Print and shaded views of the part. All mm, measured from the part's lowest x, y and z. A direction names the side the tool comes from. Round coordinates to 2 decimals unless told otherwise and drop trailing zeros. Order: outer loops, then holes, each group sorted by start corner. A loop starts at its lowest first (then second) coordinate and runs counter-clockwise, first axis right, second up. Notation, with made-up numbers: M -17.75,-14 L 18.25,-14 A17 cw 18.25,13 Z; hole C -30,40.5 d1. An arc over 180 degrees is marked long. Use CSV: the item, a comma, the result in double quotes.
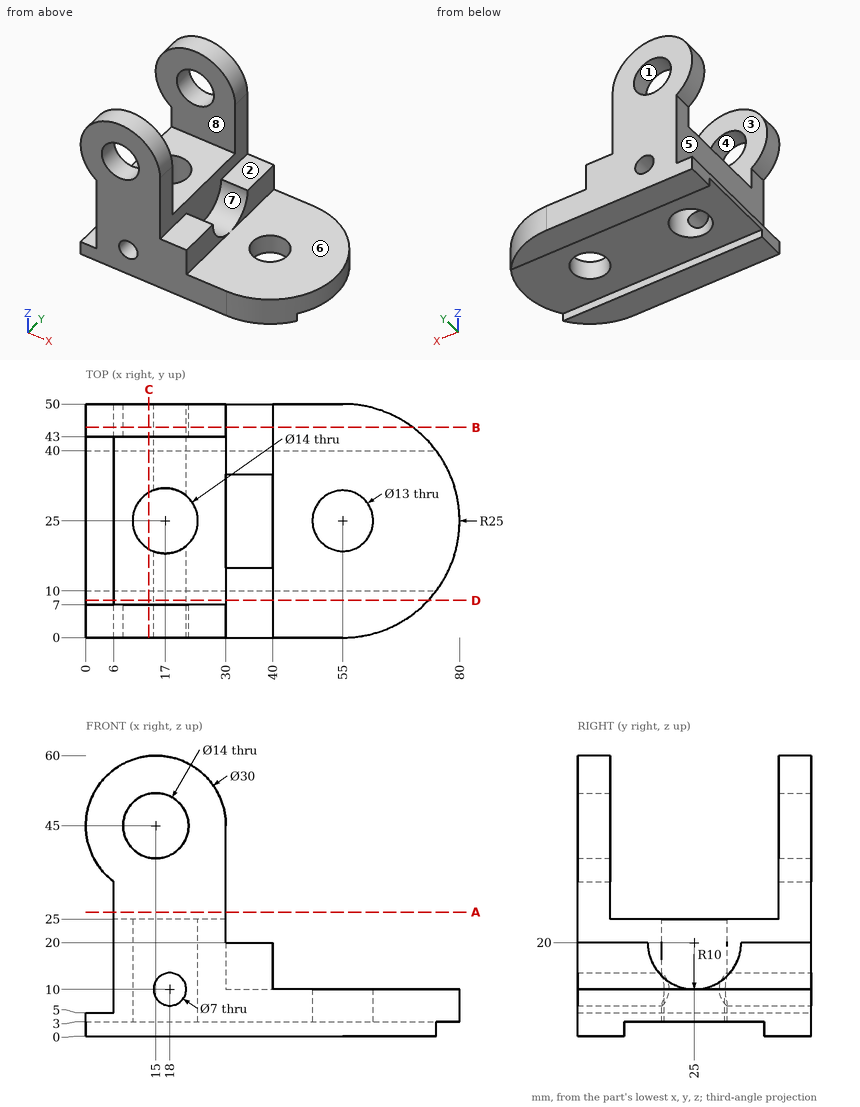
(1) Cut at D-D, the plane y = 8. Give the cut face in (x, z).
Answer block:
outline,"M 0,0 L 73.33,0 L 73.33,10 L 40,10 L 40,20 L 30,20 L 30,25 L 6,25 L 6,5 L 0,5 Z; hole C 18,10 d7"
(2) Cut at A-A, the plane z = 26.5. Give the cut face in (x, y).
Answer block:
outline,"M 6,0 L 30,0 L 30,7 L 6,7 Z; M 6,43 L 30,43 L 30,50 L 6,50 Z"
(3) Two-plate mould, pull along Z, no slides. Class the marked faces 1, 2, 3 and 4: released by +Z, released by -Z, zero draft, split by the parting line, or undercut.
Answer block:
face 1,"undercut"
face 2,"released by +Z"
face 3,"zero draft"
face 4,"undercut"
(4) Cut at C-C, the plane x = 13.5. Give the cut face in (y, z).
Answer block:
outline,"M 0,0 L 10,0 L 10,3 L 18.94,3 L 18.94,25 L 7,25 L 7,38.16 L 0,38.16 Z; M 0,51.84 L 7,51.84 L 7,59.92 L 0,59.92 Z; M 31.06,3 L 40,3 L 40,0 L 50,0 L 50,38.16 L 43,38.16 L 43,25 L 31.06,25 Z; M 43,51.84 L 50,51.84 L 50,59.92 L 43,59.92 Z"
(5) Drop flat-ended pins along their axis: pin 1 (3 mm diameter, centred on y = 13.5, z = 16, fed in from +X); pin 2 (11 mm diameter, centred on x = 32.5, y = 4.5, fed in from +Z); pin 3 (8 mm diameter, centred on y = 16, z = 24, fed in from -X). Give the stop position or say it passes through.
Answer block:
pin 1,"stops at x = 40"
pin 2,"stops at z = 54"
pin 3,"stops at x = 6"
(6) Tool access for the marked faces 5, 6, 7 and 8: list every direction of +Z, -Z, +X, -X, +Y, -Y with a clear straight run to the whole face (end or side of a thin tool).
Answer block:
face 5,"-X, +Y, -Y"
face 6,"+Z, +X, +Y, -Y"
face 7,"+Z, +X"
face 8,"+Z, +X, -X"
(7) Wall check: line 1 (X direction, y = 3, z = 45); line 2 (Z direction, x = 18, y = 35.5); line 3 (Y direction, x = 17, z = 14). Give the ranges that are in metal, low to high. Write a range as from..to.
Answer block:
line 1,"x = 0..8, 22..30"
line 2,"z = 3..6.5, 13.5..25"
line 3,"y = 0..18, 32..50"
(8) Cut at B-B, the plane y = 45. Give the cut face in (x, z).
Answer block:
outline,"M 0,0 L 70,0 L 70,10 L 40,10 L 40,20 L 30,20 L 30,45 A15 ccw long 6,33 L 6,5 L 0,5 Z; hole C 15,45 d14; hole C 18,10 d7"
